from build123d import *

# Parameters (mm, degrees)
F1_DEPTH    = 70
F2_DEPTH    = 2.5
F3_T1_DEPTH = 5
F3_T3_DEPTH = 12.6854399108
F3_T5_DEPTH = 17.5
F3_T7_DEPTH = 12.7254248594


# Not quite as in the source:
# - a fillet or chamfer that OpenCascade refuses, or shapes differently, is made with other operations: its cross-section is extruded or revolved along the edge and cut away or added


with BuildPart() as f1:
    # F0 (on Top) → F1 (new body, symmetric)
    with BuildSketch(Plane.XY):
        with BuildLine():
            ThreePointArc((2.5, -9.6824583655), (7.9056941504, -6.123724357), (10, 0))
            ThreePointArc((10, 0), (-7.0710678119, 7.0710678119), (0, -10))
            ThreePointArc((0, -10), (1.2600429248, -9.9202969627), (2.5, -9.6824583655))
        make_face()
    extrude(amount=F1_DEPTH, both=True)

    # F0 (on Top) → F2 (join, symmetric)
    with BuildSketch(Plane.XY):
        with BuildLine():
            ThreePointArc((2.5, -9.6824583655), (1.2600429248, -9.9202969627), (0, -10))
            Line((0, -10), (0, -12.4709576939))
            Line((0, -12.4709576939), (2.5, -12.4709576939))
            Line((2.5, -12.4709576939), (2.5, -9.6824583655))
        make_face()
        Polygon((2.5, -12.4709576939), (0, -12.4709576939), (0, -15), (5, -17.5), (7.5, -17.5), (7.5, -15), align=None)
    extrude(amount=F2_DEPTH, both=True)

    # F3: fillet of radius 2.5 on 4 edges, made by hand

    # F3_s2 → F3_t1 (join)
    with BuildSketch(Plane.XY.offset(-2.5)):
        with BuildLine():
            ThreePointArc((2.5, -10.9338697117), (2.8703321066, -12.2432644817), (3.871611731, -13.1647305129))
            Line((3.871611731, -13.1647305129), (2.5, -12.4709576939))
            Line((2.5, -12.4709576939), (2.5, -10.9338697117))
        make_face()
    extrude(amount=F3_T1_DEPTH)

    # F3_s4 → F3_t3 (cut)
    with BuildSketch(Plane.XY.offset(-6.3427199554)):
        with BuildLine():
            ThreePointArc((6.128388269, -14.306227181), (7.1296678934, -15.2276932122), (7.5, -16.5370879822))
            Line((7.5, -16.5370879822), (7.5, -15))
            Line((7.5, -15), (6.128388269, -14.306227181))
        make_face()
    extrude(amount=F3_T3_DEPTH, mode=Mode.SUBTRACT)

    # F3_s6 → F3_t5 (cut)
    with BuildSketch(Plane.XY.offset(-8.75)):
        with BuildLine():
            ThreePointArc((5, -17.5), (6.767766953, -16.767766953), (7.5, -15))
            Line((7.5, -15), (7.5, -17.5))
            Line((7.5, -17.5), (5, -17.5))
        make_face()
    extrude(amount=F3_T5_DEPTH, mode=Mode.SUBTRACT)

    # F3_s8 → F3_t7 (cut)
    with BuildSketch(Plane.XY.offset(-6.3627124297)):
        with BuildLine():
            ThreePointArc((0, -13.4549150281), (0.3733729791, -14.7692428084), (1.3819660113, -15.6909830056))
            Line((1.3819660113, -15.6909830056), (0, -15))
            Line((0, -15), (0, -13.4549150281))
        make_face()
    extrude(amount=F3_T7_DEPTH, mode=Mode.SUBTRACT)


solid = f1.part
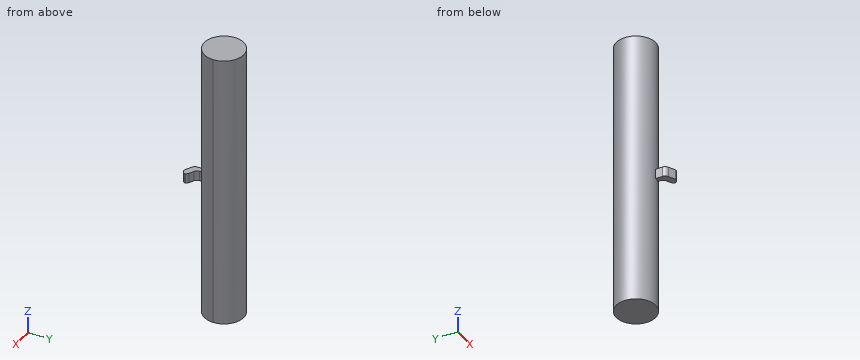
Read the model definition and answer for the solid it produces. Units are mm, in the model's axes. Coordinates: 2 decimals unless noted, no trailing zeros. Loops run counter-clockwise (first coordinate to the right, second up) from the corner with the lowest first, then second, coordinate; pieces in that order, holes last. Notation, with made-up numbers: (81.5, -27.75) - (110.5, -27.75) arc R15 cw to (110.5, -7.75) - close; hole circle Ø4 at (-7, -28.75). An arc over 180 degrees is marked (long way). Answer in a Markdown table with one row per item.
Q1. Given P1, Ø2, axis at x = -7, z = -43, coming from the +Y side; P2, Ø1.7, axis at y = -12.5, z = 0, coming from the -X side; P3, Ø12, axis at x = -5.5, z = -42.5, coming from the -Y side, each flat-ended and moving along its own axis, determine where each tip first touches the part or whether it passes through.
Here are the results:
| item | result |
|---|---|
| P1 | stops at y = 8 |
| P2 | stops at x = 0 |
| P3 | stops at y = -10 |
Q2. Find section A-A on z = -0.5. Write down the section's boundary in (x, y), plus the area to 3 significant figures.
Here are the results:
| item | result |
|---|---|
| outline | (0, -13.45) arc R2.5 ccw to (1.38, -15.69) - (5, -17.5) arc R2.5 ccw to (7.38, -15.77) arc R2.5 ccw to (6.13, -14.31) - (3.87, -13.16) arc R2.5 cw to (2.5, -10.93) - (2.5, -9.68) arc R10 ccw (long way) to (0, -10) - close |
| area | 344 mm^2 |
Q3. Find section D-D on x = -5.5. Write down the section's boundary in (y, z).
Here are the results:
| item | result |
|---|---|
| outline | (-8.35, -70) - (8.35, -70) - (8.35, 70) - (-8.35, 70) - close |
Q4. Straight lines are drawn through the part: line 1 along Z through (x, y) = (1.25, -14.25); line 2 along Y through (x, z) = (0.25, -4.5); line 3 along Y through (x, z) = (5.75, 3). For each, find the intervals that lie inside material, in ascending order. Write a range as [from, to].
Here are the results:
| item | result |
|---|---|
| line 1 | z = [-2.5, 2.5] |
| line 2 | y = [-10, 10] |
| line 3 | y = [-8.18, 8.18] |
Q5. Find section C-C on z = 24. Write down the section's boundary in (x, y), plus the area to 3 significant figures.
Here are the results:
| item | result |
|---|---|
| outline | circle Ø20 at (0, 0) |
| area | 314 mm^2 |
Q6. Find section B-B on y = -8.5. Write down the section's boundary in (x, z), plus the area to 3 significant figures.
Here are the results:
| item | result |
|---|---|
| outline | (-5.27, -70) - (5.27, -70) - (5.27, 70) - (-5.27, 70) - close |
| area | 1,470 mm^2 |
